Geometry: see drawing. Coordinates: mm, zero at the bounding-box minimum. A direction names the side the tool comes from. Coordinates: 2 decimals unless noted, no trailing zeros. Write each loop counter-clockwise with the first axis right and the second up, starting at its lowest first coordinate (ties: lowest second). Pieces come first, ordered by that corner, then holes. Notation, with made-up numbers: (-8, 66.5) - (10, 66.5) arc R23 cw to (10, 100.5) - close; hole circle Ø6 at (33.25, 3.25). An arc over 180 degrees is marked (long way). One line per question, with ' | ' between items. Start each with the question number.
1) Reachability of the marked faces 1 and 2 from +Z, -Z, +X, -X, +Y, -Y: full face, straight path, thin tool, end or side. Return the list, or none.
2) Line query: line 1 (Y direction, x = 9, z = 11.25); line 2 (Z direction, x = 6.75, y = 6.25); line 3 (Z direction, x = 7, y = 2). Output: solid intervals per line, ascending.
3) First-contact query: P1, Ø4, axis at y = 3, z = 9, coming from the +X side; P2, Ø1, axis at x = 2, z = 11.5, coming from the -Y side; P3, Ø3, axis at x = 7, z = 3, coming from the -Y side. Flat tips, straight axial feed; report the tip coordinate or a pass-through.
4) Draft query along X for the marked faces 3, 4, 5 and 6. Return one class per face: released by +X, released by -X, zero draft, split by the parting line, or undercut.
5) Section query D-D on z = 4.5. Return loops of the section in (x, y), and give its area (3 significant figures).
6) Section query A-A on z = 14.25. Return loops of the section in (x, y), and give its area (3 significant figures).
7) Section query C-C on y = 4.5. Return loops of the section in (x, z) (1 decimal), and give its area (3 significant figures).
8) Section query B-B on x = 5. Return loops of the section in (y, z), and give its area (4 significant figures).
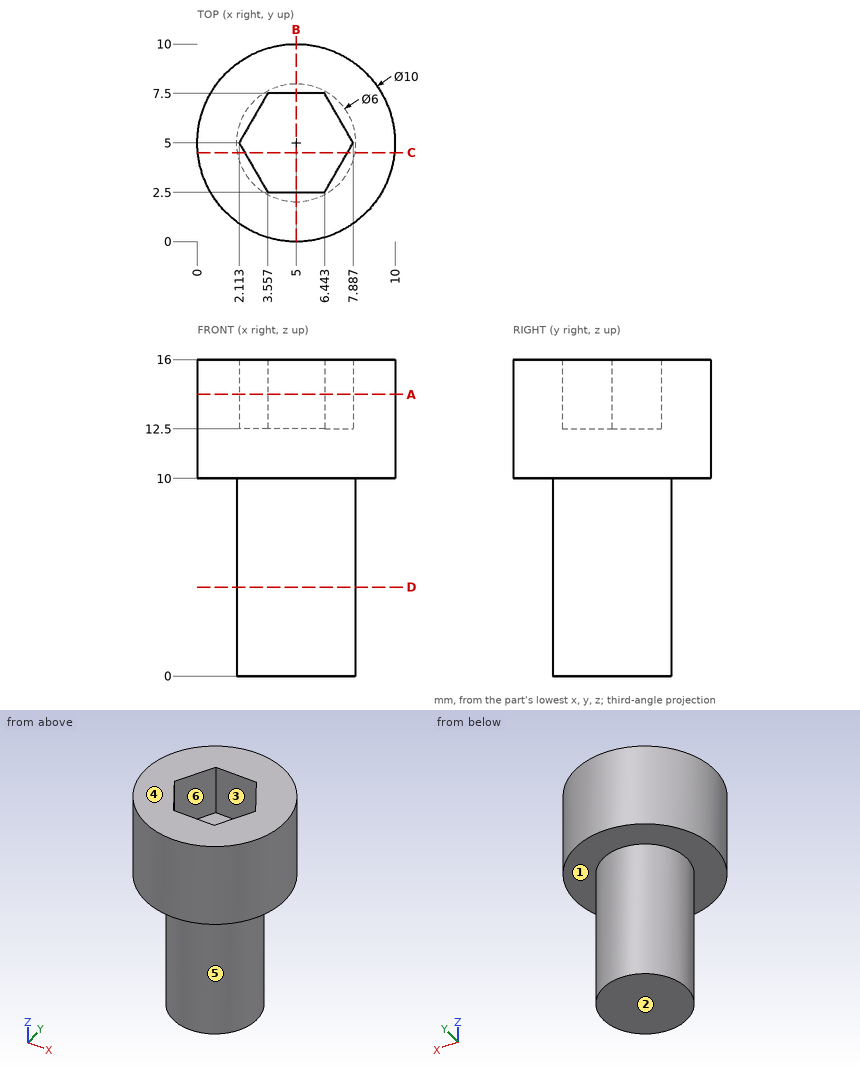
Answer key:
1) face 1: -Z | face 2: -Z, +X, -X, +Y, -Y
2) line 1: 2 to 8 | line 2: 0 to 12.5 | line 3: 10 to 16
3) P1: x = 9.99 | P2: y = 0.67 | P3: y = 2.04
4) face 3: undercut | face 4: zero draft | face 5: split by the parting line | face 6: undercut
5) outline: circle Ø6 at (5, 5) | area: 28.3 mm²
6) outline: circle Ø10 at (5, 5); hole (2.11, 5) - (3.56, 2.5) - (6.44, 2.5) - (7.89, 5) - (6.44, 7.5) - (3.56, 7.5) - close | area: 56.9 mm²
7) outline: (0, 10) - (2, 10) - (2, 0) - (8, 0) - (8, 10) - (10, 10) - (10, 16) - (7.6, 16) - (7.6, 12.5) - (2.4, 12.5) - (2.4, 16) - (0, 16) - close | area: 101 mm²
8) outline: (0, 10) - (2, 10) - (2, 0) - (8, 0) - (8, 10) - (10, 10) - (10, 16) - (7.5, 16) - (7.5, 12.5) - (2.5, 12.5) - (2.5, 16) - (0, 16) - close | area: 102.5 mm²
